Can you work these out from the model? Positions are in its coordinate system, mm. A direction names the side the tool comes from. Round coordinates to 2 decimals unless told otherwise and drop trailing zeros. Order: outer loops, then holes, each group sorted by start corner. A loop starts at its lowest first (then second) coordinate and runs counter-clockwise, first axis right, second up.
Q1. We'd pull the mould along X, two halves only. Please class faces 4 (the face through (229, 148.53, 8)), 5 (the face through (6.35, 83, 8)), 6 (the face through (113, 161.23, 8)): pulls with the +X half, pulls with the -X half, needs draft (parallel to the pull), parting line crosses it, or undercut.
Q2. If I drill on line 1 (X direction, y = 160.5, z = 8.5); line 2 (X direction, y = 52, z = 11); line 3 (Y direction, x = 184, z = 6), over which ranges is the centre line in solid material (lowest first)?
Q3. For faces 1 (the face through (234.156, 155, 8)), 2 (the face through (241, 161.23, 8)), 3 (the face through (236, 6.35, 8)), which set-ups out of +Z, -Z, +X, -X, +Y, -Y let a thin tool reach every point of the face, with its end or its side?
Q4. If we section it at C-C (z = 9.25): Count the separate pieces of the cut face and the enclosed holes in it, plus the area to 3 significant figures.
Q5. If we section it at B-B (y = 28.5): Please give me the cut outline in (x, z) (3 decimals).
Q6. Will these pins go through, and if not, where does the flat tip stop? P1, Ø3, axis at y = 154, z = 8, coming from the +X side; P2, Ø3, axis at x = 321, z = 6, coming from the -Y side; P3, Ø1.6, axis at x = 332.5, y = 125, coming from the +Z side.
Q7. If we section it at A-A (x = 128.5): Please give me the cut outline in (y, z) (3 decimals).
from build123d import *

# Parameters (mm, degrees)
F0_W     = 479.028125
F0_H     = 167.580469
F1_DEPTH = 12.7
F2_W     = 479.028125
F2_H     = 167.580469
F2_W_2   = 466.328125
F2_H_2   = 154.880469
F3_DEPTH = 9.525
F4_W     = 11.1125
F4_H     = 9.525
F5_DEPTH = 19.05
F6_R     = 1.5875
F7_DEPTH = 7.9375


with BuildPart() as f1:
    # F0 (on Top) → F1 (new body)
    with BuildSketch(Plane.XY):
        with Locations((239.514062, 83.790234)):
            Rectangle(F0_W, F0_H)
    extrude(amount=F1_DEPTH)

    # F2 (on face) → F3 (cut)
    with BuildSketch(Plane.XY.offset(12.7)):
        with Locations((239.514062, 83.790234)):
            Rectangle(F2_W, F2_H)
        with Locations((239.514062, 83.790234)):
            Rectangle(F2_W_2, F2_H_2, mode=Mode.SUBTRACT)
    extrude(amount=-F3_DEPTH, mode=Mode.SUBTRACT)

    # F4 (on face) → F5 (cut)
    with BuildSketch(Plane(origin=(0, 167.580469, 0), x_dir=(-1, 0, 0), z_dir=(0, 1, 0))):
        with Locations((-228.6, 7.9375)):
            Rectangle(F4_W, F4_H)
        with Locations((-254, 7.9375)):
            Rectangle(F4_W, F4_H)
    extrude(amount=-F5_DEPTH, mode=Mode.SUBTRACT)

    # F6 (on face) → F7 (cut)
    with BuildSketch(Plane.XY.offset(12.7)):
        with Locations((61.9125, 124.717969)):
            Circle(F6_R)
        with Locations((332.978125, 124.717969)):
            Circle(F6_R)
        with Locations((266.303125, 16.767969)):
            Circle(F6_R)
    extrude(amount=-F7_DEPTH, mode=Mode.SUBTRACT)


solid = f1.part
Solution:
1. face 4: undercut
1. face 5: pulls with the -X half
1. face 6: needs draft
2. line 1: x = 6.35 to 223.04, 234.16 to 248.44, 259.56 to 472.68
2. line 2: x = 6.35 to 472.68
2. line 3: y = 6.35 to 161.23
3. face 1: +Z, +Y
3. face 2: +Z, +X, -X, +Y
3. face 3: +Z, +X, -X, -Y
4. separate pieces: 1
4. enclosed holes: 3
4. area: 71,900 mm2
5. outline: (0, 0) - (479.028, 0) - (479.028, 3.175) - (472.678, 3.175) - (472.678, 12.7) - (6.35, 12.7) - (6.35, 3.175) - (0, 3.175) - close
6. P1: stops at x = 472.68
6. P2: stops at y = 6.35
6. P3: stops at z = 4.76
7. outline: (0, 0) - (167.58, 0) - (167.58, 3.175) - (161.23, 3.175) - (161.23, 12.7) - (6.35, 12.7) - (6.35, 3.175) - (0, 3.175) - close
